Build history of the part. All positions in model axes, mm. Face numbers are marked on the shaded views. A direction names the side the tool comes from. Coordinates: 2 decimals unless noted, no trailing zeros. Loops run counter-clockwise (first coordinate to the right, second up) from the corner with the lowest first, then second, coordinate; pieces in that order, holes last. Notation, with made-up numbers: (-28, 22) -> (17, 22) arc R21 cw to (17, 48) -> close; hole circle Ø5 at (61, 58). An arc over 180 degrees is marked (long way). One line per item, written item: value. Start each with the question number.
```python
from build123d import *

# Parameters (mm, degrees)
SKETCH1_R               = 1.995
BOSS_EXTRUDE1_DEPTH     = 33.4
SKETCH2_W               = 4.5
SKETCH2_H               = 0.920377874
CUT_EXTRUDE1_DEPTH      = 2.995
CUT_EXTRUDE1_DEPTH_BACK = 2.995
CHAMFER1_SIZE           = 0.2


with BuildPart() as part:
    # Sketch1 → Boss-Extrude1 (new body)
    with BuildSketch(Plane.XY):
        Circle(SKETCH1_R)
    extrude(amount=BOSS_EXTRUDE1_DEPTH)

    # Sketch2 → Cut-Extrude1 (cut, two sides)
    with BuildSketch(Plane(origin=(0, 0, 0), x_dir=(0, 0, -1), z_dir=(1, 0, 0))) as cut_extrude1_sk:
        with Locations((-3.75, 2.160188937)):
            Rectangle(SKETCH2_W, SKETCH2_H)
        with Locations((-3.75, -2.160188937)):
            Rectangle(SKETCH2_W, SKETCH2_H)
    extrude(amount=CUT_EXTRUDE1_DEPTH, mode=Mode.SUBTRACT)
    extrude(cut_extrude1_sk.sketch, amount=-CUT_EXTRUDE1_DEPTH_BACK, mode=Mode.SUBTRACT)

    # Chamfer1
    chamfer1_edges = [part.edges().sort_by_distance(p)[0] for p in [
        (-1.995, 0, 0),
        (-1.995, 0, 33.4),
    ]]
    chamfer(chamfer1_edges, length=CHAMFER1_SIZE)


solid = part.part
```
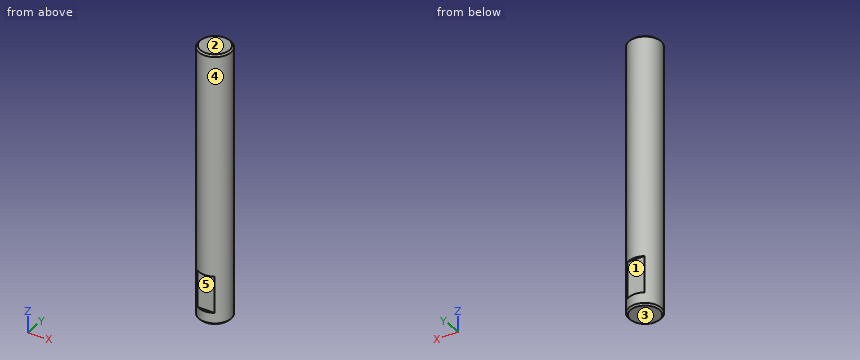
Item 1: Probe probe 1 along Y at (x, z) = (-0.85, 7.5); probe 2 along Y at (x, z) = (1.75, 19); probe 3 along X at (y, z) = (0.4, 19). List the from-to ranges inside material, lowest first.
Item 2: Two-plate mould, pull along Z, no slides. Class the marked faces 3, 4 and 5: +Z half, -Z half, draft (parallel to the pull), parting line (faces both ways), or undercut.
Item 3: Tool access for the marked faces 1 and 2: list every direction of +Z, -Z, +X, -X, +Y, -Y with a clear straight run to the whole face (end or side of a thin tool).
Item 4: Band-saw the part on B-B, the plane z = 9. List the corners of the cut face in (x, y) (3 decimals).
Item 5: Drop flat-ended pins along their axis: pin 1 Ø0.6 at (x, z) = (0.5, 4.5) entering from +Y; pin 2 Ø1.7 at (x, z) = (-0.5, 3) entering from -Y. Give the stop position or say it passes through.
Item 6: Band-saw the part on A-A, the plane x = 0. List the corners of the cut face in (y, z) (3 decimals), and give its area (3 significant figures).
Item 7: Band-saw the part on C-C, the plane z = 3. List the corners of the cut face in (x, y) (3 decimals), and give its area (3 significant figures).
Worked out:
1. probe 1: y = -1.8 to 1.8
1. probe 2: y = -0.96 to 0.96
1. probe 3: x = -1.95 to 1.95
2. face 3: -Z half
2. face 4: draft
2. face 5: undercut
3. face 1: +X, -X, +Y
3. face 2: +Z, +X, -X, +Y, -Y
4. outline: circle Ø3.99 at (0, 0)
5. pin 1: stops at y = 1.7
5. pin 2: stops at y = -1.7
6. outline: (-1.995, 0.2) -> (-1.795, 0) -> (1.795, 0) -> (1.995, 0.2) -> (1.995, 1.5) -> (1.7, 1.5) -> (1.7, 6) -> (1.995, 6) -> (1.995, 33.2) -> (1.795, 33.4) -> (-1.795, 33.4) -> (-1.995, 33.2) -> (-1.995, 6) -> (-1.7, 6) -> (-1.7, 1.5) -> (-1.995, 1.5) -> close
6. area: 131 mm²
7. outline: (-1.044, -1.7) -> (1.044, -1.7) arc R1.995 ccw to (1.044, 1.7) -> (-1.044, 1.7) arc R1.995 ccw to start
7. area: 11.7 mm²
